Here's how the part is built. I have some questions about the finished solid (model axes, mm). Face numbers are marked on the shaded views. A direction names the side the tool comes from. Round coordinates to 2 decimals unless told otherwise and drop trailing zeros. Order: outer loops, then holes, each group sorted by start corner. A loop starts at its lowest first (then second) coordinate and runs counter-clockwise, first axis right, second up.
```python
from build123d import *

# Parameters (mm, degrees)
F0_R     = 51
F1_DEPTH = 42.5
F2_R     = 5
F3_DEPTH = 25
F4_R     = 17.5
F5_R     = 24.5
F6_DEPTH = 17.8
F7_R     = 1


with BuildPart() as f1:
    # F0 (on Top) → F1 (new body)
    with BuildSketch(Plane.XY):
        Circle(F0_R)
    extrude(amount=F1_DEPTH)

    # F2 (on Top) → F3 (cut)
    with BuildSketch(Plane.XY):
        with Locations((0, -35)):
            Circle(F2_R)
        with Locations((30.310889, -17.5)):
            Circle(F2_R)
        with Locations((30.310889, 17.5)):
            Circle(F2_R)
        with Locations((0, 35)):
            Circle(F2_R)
        with Locations((-30.310889, 17.5)):
            Circle(F2_R)
        with Locations((-30.310889, -17.5)):
            Circle(F2_R)
        Circle(F2_R)
    extrude(amount=F3_DEPTH, mode=Mode.SUBTRACT)

    # F4
    f4_edges = [f1.edges().sort_by_distance(p)[0] for p in [
        (-51, 0, 42.5),
    ]]
    fillet(f4_edges, radius=F4_R)

    # F5 (on face) → F6 (join)
    with BuildSketch(Plane.XY.offset(42.5)):
        Circle(F5_R)
    extrude(amount=F6_DEPTH)

    # F7
    f7_edges = [f1.edges().sort_by_distance(p)[0] for p in [
        (-24.5, 0, 60.3),
    ]]
    fillet(f7_edges, radius=F7_R)


solid = f1.part
```
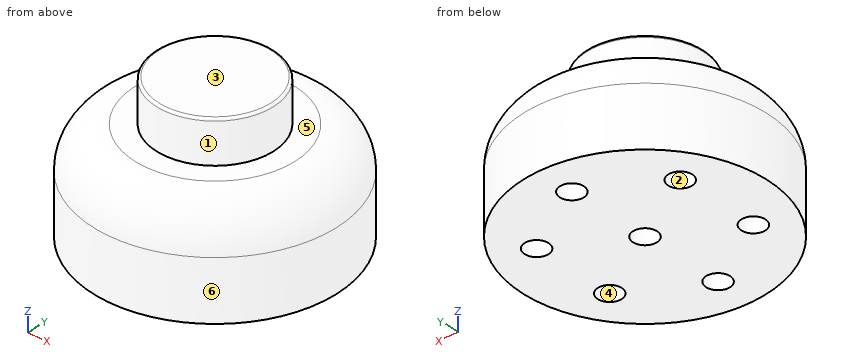
1. If we section it at A-A, the plane z = 5: Write out the boundary of the cut face in (x, y).
Evaluation:
outline: circle Ø102 at (0, 0); hole circle Ø10 at (-30.31, -17.5); hole circle Ø10 at (-30.31, 17.5); hole circle Ø10 at (0, -35); hole circle Ø10 at (0, 0); hole circle Ø10 at (0, 35); hole circle Ø10 at (30.31, -17.5); hole circle Ø10 at (30.31, 17.5)
2. On a 3-axis mill with a long thin cutter (end or side, diameter ignored), from which of +Z, -Z, +X, -X, +Y, -Y can I reach the whole of each face in a straight line? I mean the marked faces 4, 5 and 6. Say none if no direction works.
Evaluation:
face 4: -Z
face 5: +Z
face 6: +Z, -Z
3. If we mould it in two halves opening along Y, with no side actions, what happens to the marked faces 1, 2 and 3? For each: released by +Y, released by -Y, zero draft, split by the parting line, or undercut.
Evaluation:
face 1: split by the parting line
face 2: undercut
face 3: zero draft
4. If we section it at C-C, the plane x = 0: Write out the boundary of the cut face in (y, z), and give its area (3 significant figures).
Evaluation:
outline: (-51, 0) - (-40, 0) - (-40, 25) - (-30, 25) - (-30, 0) - (-5, 0) - (-5, 25) - (5, 25) - (5, 0) - (30, 0) - (30, 25) - (40, 25) - (40, 0) - (51, 0) - (51, 25) arc R17.5 ccw to (33.5, 42.5) - (24.5, 42.5) - (24.5, 59.3) arc R1 ccw to (23.5, 60.3) - (-23.5, 60.3) arc R1 ccw to (-24.5, 59.3) - (-24.5, 42.5) - (-33.5, 42.5) arc R17.5 ccw to (-51, 25) - close
area: 4,330 mm2
5. I'm going to push flat-ended pins straight in: P1, Ø2, axis at x = -32, y = -21.5, coming from the -Z side; P2, Ø6, axis at x = -13, z = 29.5, coming from the -Y side; P3, Ø3, axis at x = 28, y = -17.5, coming from the -Z side; P4, Ø6, axis at x = 30.31, y = 17.5, coming from the +Z side. Where does each tip first touch, or does it pass through?
Evaluation:
P1: stops at z = 0
P2: stops at y = -49.67
P3: stops at z = 25
P4: stops at z = 42.5
6. If we section it at B-B, the plane y = 0: Write out the boundary of the cut face in (x, z).
Evaluation:
outline: (-51, 0) - (-5, 0) - (-5, 25) - (5, 25) - (5, 0) - (51, 0) - (51, 25) arc R17.5 ccw to (33.5, 42.5) - (24.5, 42.5) - (24.5, 59.3) arc R1 ccw to (23.5, 60.3) - (-23.5, 60.3) arc R1 ccw to (-24.5, 59.3) - (-24.5, 42.5) - (-33.5, 42.5) arc R17.5 ccw to (-51, 25) - close
7. I need wall thicknesses on probe 1 along Y at (x, z) = (0, 15.5); probe 2 along X at (y, z) = (-17, 18); probe 3 along Y at (x, z) = (-34.5, 22). Which ranges of each line are inside material? Lowest first, please.
Evaluation:
probe 1: y = -51 to -40, -30 to -5, 5 to 30, 40 to 51
probe 2: x = -48.08 to -35.29, -25.34 to 25.34, 35.29 to 48.08
probe 3: y = -37.56 to -20.23, -14.77 to 14.77, 20.23 to 37.56
8. If we section it at D-D, the plane z = 35.5: Write out the boundary of the cut face in (x, y).
Evaluation:
outline: circle Ø95 at (0, 0)
